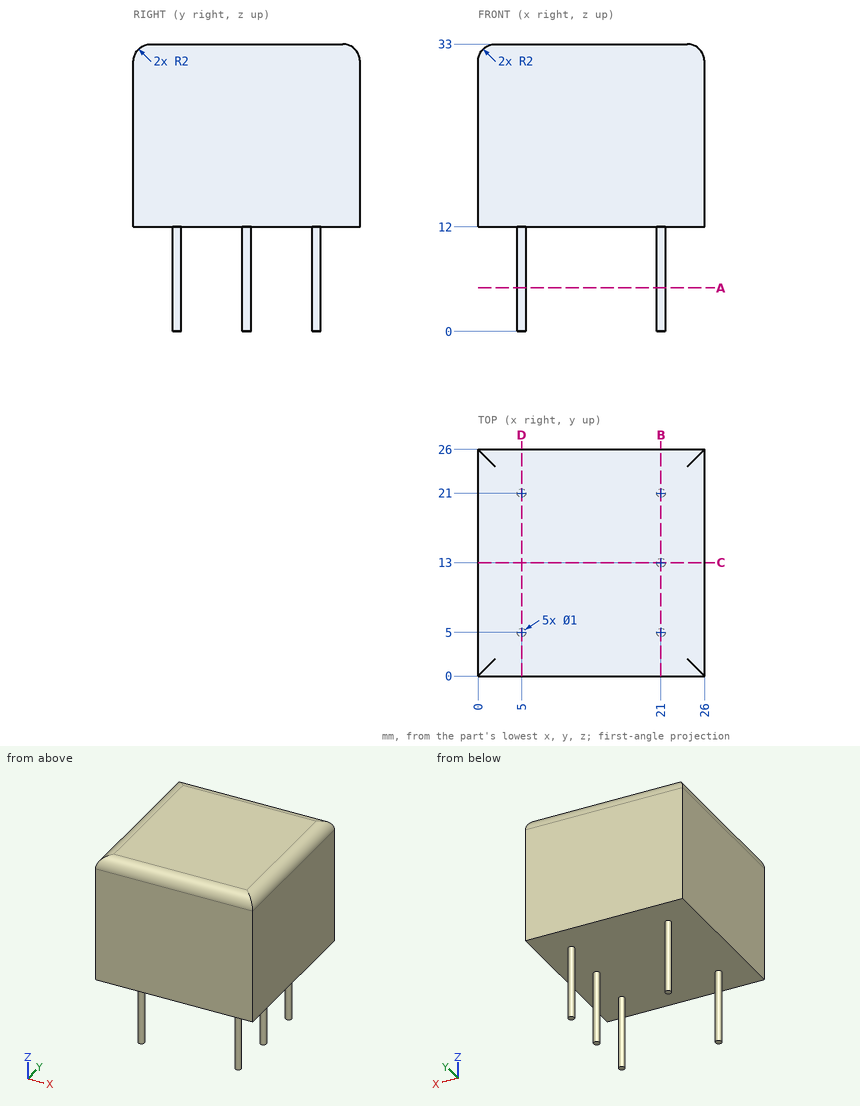
Geometry: see drawing. Coordinates: mm, zero at the bounding-box minimum. Round coordinates to 2 decimals unless told otherwise and drop trailing zeros. Write each loop counter-clockwise with the first axis right and the second up, starting at its lowest first coordinate (ties: lowest second). Pieces come first, ordered by that corner, then holes.
1) Cut plane D-D (x = 5). Return the cut outline in (y, z).
2) Cut plane B-B (x = 21). Return the cut outline in (y, z).
3) Contact query for flat-ended pins moving along their axis: P1, Ø4, axis at x = 12.5, z = 8.5, coming from the -Y side; P2, Ø10, axis at y = 12, z = 11.5, coming from the +X side; P3, Ø1.5, axis at x = 21.5, y = 18.5, coming from the -Z side. Output: stop coordinate, or through.
4) Ray query, L1, parallel to Z at x = 15.5, y = 3.5; L2, parallel to Z at x = 5.5, y = 24.75. Return the intervals inside material, ascending.
5) Cut plane A-A (z = 5). Return the cut outline in (x, y), then the cut area to 3 significant figures.
6) Cut plane C-C (y = 13). Return the cut outline in (x, z).
Geometry says:
1. outline: (0, 12) - (4.5, 12) - (4.5, 0) - (5.5, 0) - (5.5, 12) - (20.5, 12) - (20.5, 0) - (21.5, 0) - (21.5, 12) - (26, 12) - (26, 31) arc R2 ccw to (24, 33) - (2, 33) arc R2 ccw to (0, 31) - close
2. outline: (0, 12) - (4.5, 12) - (4.5, 0) - (5.5, 0) - (5.5, 12) - (12.5, 12) - (12.5, 0) - (13.5, 0) - (13.5, 12) - (20.5, 12) - (20.5, 0) - (21.5, 0) - (21.5, 12) - (26, 12) - (26, 31) arc R2 ccw to (24, 33) - (2, 33) arc R2 ccw to (0, 31) - close
3. P1: passes through
3. P2: stops at x = 26
3. P3: stops at z = 12
4. L1: z = 12 to 33
4. L2: z = 12 to 32.85
5. outline: circle Ø1 at (5, 5); circle Ø1 at (5, 21); circle Ø1 at (21, 5); circle Ø1 at (21, 13); circle Ø1 at (21, 21)
5. area: 3.93 mm2
6. outline: (0, 12) - (20.5, 12) - (20.5, 0) - (21.5, 0) - (21.5, 12) - (26, 12) - (26, 31) arc R2 ccw to (24, 33) - (2, 33) arc R2 ccw to (0, 31) - close
